Build history of the part. All positions in model axes, mm. A direction names the side the tool comes from. Round coordinates to 2 decimals unless told otherwise and drop trailing zeros. Order: outer loops, then holes, each group sorted by start corner. A loop starts at its lowest first (then second) coordinate and runs counter-clockwise, first axis right, second up. Notation, with made-up numbers: (59, 85) -> (108, 85) arc R25 cw to (108, 119) -> close; hole circle Ø4 at (-23, 34). An arc over 180 degrees is marked (long way). Answer as a JSON object with one key per item and string values.
from build123d import *

# Parameters (mm, degrees)
SKETCH4_W           = 413.09178157
SKETCH4_H           = 413.09178157
BOSS_EXTRUDE3_DEPTH = 6.604
SKETCH6_R           = 77.79258
CUT_EXTRUDE1_DEPTH  = 6.604
CUT_EXTRUDE2_DEPTH  = 6.604
CUT_EXTRUDE3_DEPTH  = 6.604


with BuildPart() as part:
    # Sketch4 → Boss-Extrude3 (new body)
    with BuildSketch(Plane(origin=(0, 0, 0), x_dir=(1, 0, 0), z_dir=(0, 1, 0))):
        Rectangle(SKETCH4_W, SKETCH4_H)
    extrude(amount=BOSS_EXTRUDE3_DEPTH)

    # Sketch6 → Cut-Extrude1 (cut)
    with BuildSketch(Plane(origin=(0, 6.604, 0), x_dir=(1, 0, 0), z_dir=(0, 1, 0))):
        Circle(SKETCH6_R)
    extrude(amount=-CUT_EXTRUDE1_DEPTH, mode=Mode.SUBTRACT)

    # Sketch8 → Cut-Extrude2 (cut)
    with BuildSketch(Plane(origin=(0, 6.604, 0), x_dir=(1, 0, 0), z_dir=(0, 1, 0))):
        Polygon((-174.055324139, -169.457433005), (169.457433005, 174.055324139), (174.055324139, 169.457433005), (-169.457433005, -174.055324139), align=None)
    extrude(amount=-CUT_EXTRUDE2_DEPTH, mode=Mode.SUBTRACT)

    # Sketch9 → Cut-Extrude3 (cut)
    with BuildSketch(Plane(origin=(0, 6.604, 0), x_dir=(1, 0, 0), z_dir=(0, 1, 0))):
        Polygon((174.064304395, -169.448452748), (-169.448452748, 174.064304395), (-174.064304395, 169.448452748), (169.448452748, -174.064304395), align=None)
    extrude(amount=-CUT_EXTRUDE3_DEPTH, mode=Mode.SUBTRACT)


solid = part.part
1) Cut at A-A, the plane z = -17.5. Give the cut face in (x, y), plus the area to 3 significant figures.
Checked values:
{"outline": "(-206.55, 0) -> (-75.8, 0) -> (-75.8, 6.6) -> (-206.55, 6.6) -> close; (75.8, 0) -> (206.55, 0) -> (206.55, 6.6) -> (75.8, 6.6) -> close", "area": "1,730 mm²"}
2) Pull direction Z, two halves, no side cores. Call faces 3 (the face through (110.2, 3.3, -114.8)), 4 (the face through (89, 0, -3)): pulls with the +Z half, pulls with the -Z half, needs draft (parallel to the pull), parting line crosses it, or undercut.
Checked values:
{"face 3": "undercut", "face 4": "needs draft"}
3) Cut at B-B, the plane y = 4.5. Give the cut face in (x, z), plus the area to 3 significant figures.
Checked values:
{"outline": "(-206.55, -206.55) -> (206.55, -206.55) -> (206.55, 206.55) -> (-206.55, 206.55) -> close; hole (-174.06, -169.45) -> (-169.45, -174.06) -> (-52.65, -57.27) arc R77.79 ccw to (52.66, -57.26) -> (169.46, -174.06) -> (174.06, -169.46) -> (57.26, -52.66) arc R77.79 ccw to (57.27, 52.65) -> (174.06, 169.45) -> (169.45, 174.06) -> (52.65, 57.27) arc R77.79 ccw to (-52.66, 57.26) -> (-169.46, 174.06) -> (-174.06, 169.46) -> (-57.26, 52.66) arc R77.79 ccw to (-57.27, -52.65) -> close", "area": "147,000 mm²"}
4) Which spindle directions (+Z, -Z, +X, -X, +Y, -Y) get a long thin tool onto all of the face, cutting with end or side? Do faces 1 (the face through (116.5, 3.3, -111.9)), 2 (the face through (89, 6.604, -3)). Say none if no direction does.
Checked values:
{"face 1": "+Y, -Y", "face 2": "+Z, -Z, +X, -X, +Y"}
5) Cut at C-C, the plane x = -163.5. Give the cut face in (y, z), plus the area to 3 significant figures.
Checked values:
{"outline": "(0, -206.55) -> (6.6, -206.55) -> (6.6, -168.12) -> (0, -168.12) -> close; (0, -158.88) -> (6.6, -158.88) -> (6.6, 158.9) -> (0, 158.9) -> close; (0, 168.1) -> (6.6, 168.1) -> (6.6, 206.55) -> (0, 206.55) -> close", "area": "2,610 mm²"}
6) Probe L1, parallel to Z at x = -86, y = 4; L2, parallel to X at y = 3, z = 122; L3, parallel to Z at x = -132, y = 2.75. List the from-to ranges inside material, lowest first. Write a range as from..to.
Checked values:
{"L1": "z = -206.55..-90.62, -81.38..81.4, 90.6..206.55", "L2": "x = -206.55..-126.6, -117.4..117.38, 126.62..206.55", "L3": "z = -206.55..-136.62, -127.38..127.4, 136.6..206.55"}
7) Cut at D-D, the plane x = -70.5. Give the cut face in (y, z), plus the area to 3 significant figures.
Checked values:
{"outline": "(0, -206.55) -> (6.6, -206.55) -> (6.6, -75.12) -> (0, -75.12) -> close; (0, -65.88) -> (6.6, -65.88) -> (6.6, -32.89) -> (0, -32.89) -> close; (0, 32.89) -> (6.6, 32.89) -> (6.6, 65.9) -> (0, 65.9) -> close; (0, 75.1) -> (6.6, 75.1) -> (6.6, 206.55) -> (0, 206.55) -> close", "area": "2,170 mm²"}
8) Flat gauge pin, fed straight in: pin 1 Ø6 at (x, z) = (149.5, 44) entering from -Y. Where does the tip first touch, or does it go through?
Checked values:
{"pin 1": "stops at y = 0"}
